Design review of the part shown in the three views and the two pictorial views. Dimensions are in mm from the part's minimum x, y and z. A direction names the side the tool comes from. Coordinates: 2 decimals unless noted, no trailing zeros. Loops run counter-clockwise (first coordinate to the right, second up) from the corner with the lowest first, then second, coordinate; pieces in that order, holes last. Notation, with made-up numbers: (-25, 62) -> (7, 62) arc R24 ccw to (7, 97) -> close; hole circle Ø9 at (-29.5, 15). An arc over 180 degrees is marked (long way). One line per item, written item: value.
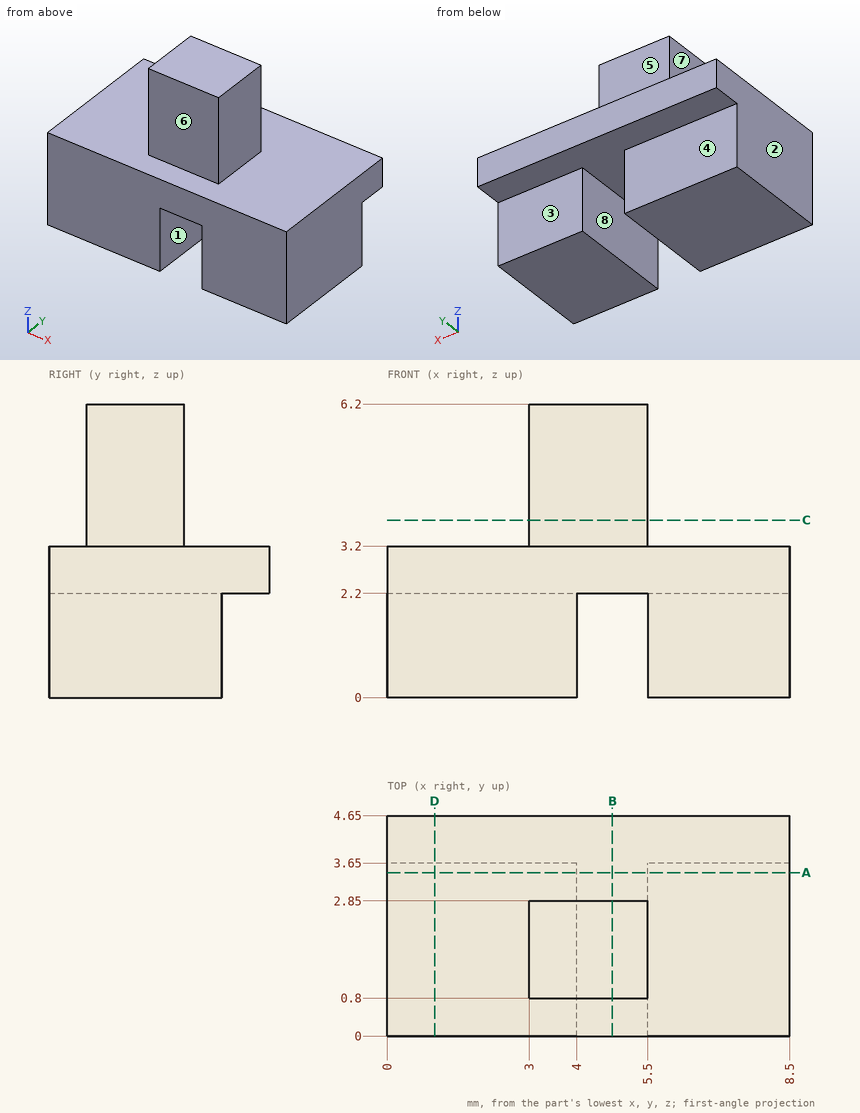
1. For the marked faces 4, 5, 6, 7 and 8, list the 3-axis set-ups (+Z, -Z, +X, -X, +Y, -Y) from which the entire face can be reached by the end or side of a thin tool; tool diameter is ignored.
Return value:
face 4: -Z, +X, -X, +Y
face 5: +Z, +X, -X, +Y
face 6: +Z, +X, -X, -Y
face 7: +Z, -X, +Y, -Y
face 8: -Z, +Y, -Y
2. Take a section at A-A, the plane y = 3.45. Give the boundary of the cut face in (x, z), and give its area (3 significant figures).
Return value:
outline: (0, 0) -> (4, 0) -> (4, 2.2) -> (5.5, 2.2) -> (5.5, 0) -> (8.5, 0) -> (8.5, 3.2) -> (0, 3.2) -> close
area: 23.9 mm2
3. Take a section at D-D, the plane x = 1. Give the boundary of the cut face in (y, z), and give its area (3 significant figures).
Return value:
outline: (0, 0) -> (3.65, 0) -> (3.65, 2.2) -> (4.65, 2.2) -> (4.65, 3.2) -> (0, 3.2) -> close
area: 12.7 mm2
4. Take a section at C-C, the plane z = 3.75. Give the boundary of the cut face in (x, y).
Return value:
outline: (3, 0.8) -> (5.5, 0.8) -> (5.5, 2.85) -> (3, 2.85) -> close
5. To check wall thickness, follow probe 1 along X at (y, z) = (3.15, 1.25); probe 2 along Z at (x, y) = (5, 0.55); probe 3 along X at (y, z) = (1.8, 4.25). State the ranges of each line that lie inside material, in increasing order. Write a range as from..to.
Return value:
probe 1: x = 0..4, 5.5..8.5
probe 2: z = 2.2..3.2
probe 3: x = 3..5.5
6. Insertion check: pin 1 Ø1.1 at (x, z) = (2.5, 0.5) entering from +Y; pin 2 Ø1.2 at (x, z) = (4.5, 4.5) entering from +Y; pin 3 Ø2 at (x, z) = (4, 5) entering from -Y. Each pin has a flat end and moves straight along its axis. Give the tip position at first contact, or say it passes through.
Return value:
pin 1: stops at y = 3.65
pin 2: stops at y = 2.85
pin 3: stops at y = 0.8
7. Take a section at B-B, the plane x = 4.75. Give the boundary of the cut face in (y, z).
Return value:
outline: (0, 2.2) -> (4.65, 2.2) -> (4.65, 3.2) -> (2.85, 3.2) -> (2.85, 6.2) -> (0.8, 6.2) -> (0.8, 3.2) -> (0, 3.2) -> close
8. The part is to be moulded in two halves that separate along X. For the marked faces 1, 2 and 3, say which applies: pulls with the +X half, pulls with the -X half, needs draft (parallel to the pull), parting line crosses it, or undercut.
Return value:
face 1: undercut
face 2: pulls with the -X half
face 3: needs draft
